```python
from build123d import *

# Parameters (mm, degrees)
BOSS_EXTRUDE2_DEPTH = 4.445


with BuildPart() as part:
    # Sketch1 → Boss-Extrude2 (new body)
    with BuildSketch(Plane(origin=(0, 0, 0), x_dir=(1, 0, 0), z_dir=(0, 1, 0))):
        with BuildLine():
            Line((-51.06889371, 4.150009473), (-51.06889371, 64.857309497))
            ThreePointArc((-51.06889371, 64.857309497), (0, 82.55), (51.06889371, 64.857309497))
            Line((51.06889371, 64.857309497), (51.06889371, 4.150009473))
            Line((51.06889371, 4.150009473), (19.05, 4.150009473))
            Line((19.05, 4.150009473), (19.05, 14.2875))
            Line((19.05, 14.2875), (19.05, 18.374009473))
            Line((19.05, 18.374009473), (-19.05, 18.374009473))
            Line((-19.05, 18.374009473), (-19.05, 14.2875))
            Line((-19.05, 14.2875), (-19.05, 4.150009473))
            Line((-19.05, 4.150009473), (-51.06889371, 4.150009473))
        make_face()
    extrude(amount=BOSS_EXTRUDE2_DEPTH)


solid = part.part
```
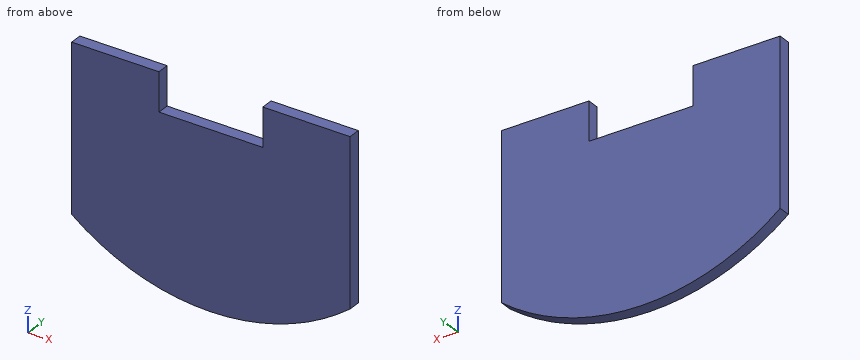
Source: CAD feature listing. Evaluate the final solid. Frame: model axes, mm. Round coordinates to 2 decimals unless told otherwise and drop trailing zeros. Loops run counter-clockwise (first coordinate to the right, second up) from the corner with the lowest first, then second, coordinate; pieces in that order, holes last. Notation, with made-up numbers: M 68.25,48 L 126.25,48 A21 cw 126.25,68 Z; hole C 29,78 d9. An arc over 180 degrees is marked long. Use a Markdown table: item, result. Add a question column.
1. Ray query, line 1 along X through (y, z) = (3.4, -12.5); line 2 along Z through (x, y) = (43.5, 1.6); line 3 along Z through (x, y) = (-28.5, 3.55). Return the intervals inside material, ascending. Write a range as [from, to].
2. Cut plane B-B, the plane x = 0.5. Output: boundary loops of the cut face in (y, z) (3 decimals), and give its area (3 significant figures).
3. Cut plane A-A, the plane y = 2.25. Output: boundary loops of the cut face in (x, z), and give its area (3 significant figures).
4. Cut plane C-C, the plane z = -75. Output: boundary loops of the cut face in (x, y) (3 decimals), and give its area (3 significant figures).
Solution:
| question | item | result |
|---|---|---|
| 1 | line 1 | x = [-51.07, -19.05], [19.05, 51.07] |
| 1 | line 2 | z = [-70.16, -4.15] |
| 1 | line 3 | z = [-77.47, -4.15] |
| 2 | outline | M 0,-82.548 L 4.445,-82.548 L 4.445,-18.374 L 0,-18.374 Z |
| 2 | area | 285 mm2 |
| 3 | outline | M -51.07,-64.86 A82.55 ccw 51.07,-64.86 L 51.07,-4.15 L 19.05,-4.15 L 19.05,-18.37 L -19.05,-18.37 L -19.05,-4.15 L -51.07,-4.15 Z |
| 3 | area | 6,890 mm2 |
| 4 | outline | M -34.489,0 L 34.489,0 L 34.489,4.445 L -34.489,4.445 Z |
| 4 | area | 307 mm2 |
